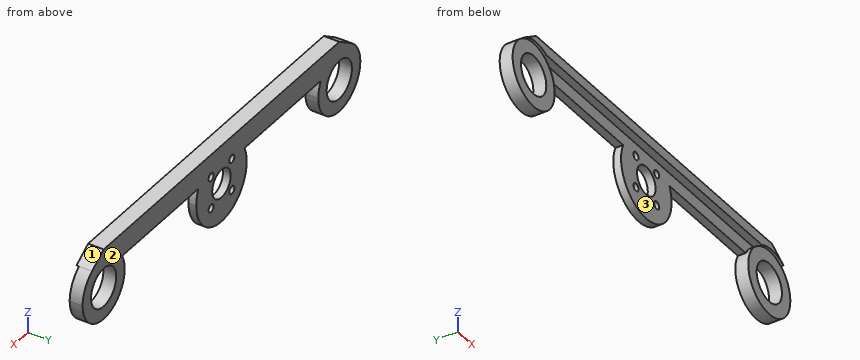
```python
from build123d import *

# Parameters (mm, degrees)
F0_R     = 1.5
F0_R_2   = 5.5
F1_DEPTH = 3
F0_R_3   = 7.5
F2_DEPTH = 5
F4_DEPTH = 3


with BuildPart() as f1:
    # F0 (on Front) → F1 (new body)
    with BuildSketch(Plane.XZ):
        with BuildLine():
            ThreePointArc((15, 0), (14.683594694, 3.0646446553), (13.7477270849, 6))
            ThreePointArc((13.7477270849, 6), (8.2158383626, 12.549900398), (0, 15))
            ThreePointArc((0, 15), (-8.2158383626, 12.549900398), (-13.7477270849, 6))
            ThreePointArc((-13.7477270849, 6), (-3.0646446553, -14.683594694), (15, 0))
        make_face()
        with Locations((-6.1518289963, -6.1518289963)):
            Circle(F0_R, mode=Mode.SUBTRACT)
        with Locations((6.1518289963, -6.1518289963)):
            Circle(F0_R, mode=Mode.SUBTRACT)
        with Locations((-6.1518289963, 6.1518289963)):
            Circle(F0_R, mode=Mode.SUBTRACT)
        Circle(F0_R_2, mode=Mode.SUBTRACT)
        with Locations((6.1518289963, 6.1518289963)):
            Circle(F0_R, mode=Mode.SUBTRACT)
        with BuildLine():
            ThreePointArc((59.0341439003, 6), (67.0016723737, 12.135074431), (76.9096349799, 10.4166666667))
            Line((76.9096349799, 10.4166666667), (70, 15))
            Line((70, 15), (0, 15))
            ThreePointArc((0, 15), (8.2158383626, 12.549900398), (13.7477270849, 6))
            Line((13.7477270849, 6), (59.0341439003, 6))
        make_face()
        with BuildLine():
            ThreePointArc((-13.7477270849, 6), (-8.2158383626, 12.549900398), (0, 15))
            Line((0, 15), (-70, 15))
            Line((-70, 15), (-76.9096349799, 10.4166666667))
            ThreePointArc((-76.9096349799, 10.4166666667), (-67.0016723737, 12.135074431), (-59.0341439003, 6))
            Line((-59.0341439003, 6), (-13.7477270849, 6))
        make_face()
    extrude(amount=F1_DEPTH)

    # F0 (on Front) → F2 (join)
    with BuildSketch(Plane.XZ):
        with BuildLine():
            ThreePointArc((59.0341439003, 6), (66.9034859315, -12.1103922572), (82.5, 0))
            ThreePointArc((82.5, 0), (81.0140918202, 5.9109881894), (76.9096349799, 10.4166666667))
            ThreePointArc((76.9096349799, 10.4166666667), (67.0016723737, 12.135074431), (59.0341439003, 6))
        make_face()
        with Locations((70, 0)):
            Circle(F0_R_3, mode=Mode.SUBTRACT)
        with BuildLine():
            ThreePointArc((-57.5, 0), (-57.8896077428, 3.0965140685), (-59.0341439003, 6))
            ThreePointArc((-59.0341439003, 6), (-67.0016723737, 12.135074431), (-76.9096349799, 10.4166666667))
            ThreePointArc((-76.9096349799, 10.4166666667), (-75.9109881894, -11.0140918202), (-57.5, 0))
        make_face()
        with Locations((-70, 0)):
            Circle(F0_R_3, mode=Mode.SUBTRACT)
    extrude(amount=F2_DEPTH)

    # F3 (on face) → F4 (join)
    with BuildSketch(Plane.XZ.offset(3)):
        with BuildLine():
            Line((0, 11), (64.0628289565, 11))
            ThreePointArc((64.0628289565, 11), (70.5670017384, 12.4871337395), (76.9096349799, 10.4166666667))
            Line((76.9096349799, 10.4166666667), (70, 15))
            Line((70, 15), (-70, 15))
            Line((-70, 15), (-76.9096349799, 10.4166666667))
            ThreePointArc((-76.9096349799, 10.4166666667), (-70.5670017384, 12.4871337395), (-64.0628289565, 11))
            Line((-64.0628289565, 11), (0, 11))
        make_face()
    extrude(amount=F4_DEPTH)


solid = f1.part
```
Can you work these out from the model? Positions are in its coordinate system, mm. Face numbers are marked on the shaded views. Give positions to 0.01 mm unless a question says otherwise; leave off trailing zeros. Order: outer loops, then holes, each group sorted by start corner. A loop starts at its lowest first (then second) coordinate and runs counter-clockwise, first axis right, second up. Notation, with made-up numbers: M 73.5,89 L 84.5,89 A21 cw 84.5,112 Z; hole C 45.25,43 d9. An arc over 180 degrees is marked long. Write item = value, one per line. Start each with the question number.
Q1. Suppose I cut it at A-A (x = 0). Write out the boundary of the cut face in (y, z), plus the area to 3 significant figures.
Q2. Suppose I cut it at D-D (z = -11). Write out the boundary of the cut face in (x, y).
Q3. We'd pull the mould along X, two halves only. Please class the marked faces 1, 2 and 3: pulls with the +X half, pulls with the -X half, needs draft (parallel to the pull), parting line crosses it, or undercut.
Q4. Will these pins go through, and if not, where does the flat tip stop? pin 1 Ø2.5 at (x, y) = (9, -4.5) entering from -Z; pin 2 Ø2 at (y, z) = (-2, -8) entering from -X; pin 3 Ø2.5 at (x, y) = (41.5, -1) entering from -Z; pin 4 Ø1.8 at (x, z) = (6.15, 6.15) entering from -Y (3 decimals).
Q5. Suppose I cut it at B-B (z = -3). Write out the boundary of the cut face in (x, y).
Q6. I need wall thicknesses on probe 1 along X at (y, z) = (-1.9, 0.5); probe 2 along Z at (x, y) = (-70, -2.25); probe 3 along X at (y, z) = (-0.9, -11.5). Which ranges of each line are inside material? Lowest first, please. Write a range as [from, to].
Q7. Suppose I cut it at C-C (x = -41.5). Write out the boundary of the cut face in (y, z).
Check result:
q1.outline = M -6,11 L -3,11 L -3,5.5 L 0,5.5 L 0,15 L -6,15 Z; M -3,-15 L 0,-15 L 0,-5.5 L -3,-5.5 Z
q1.area = 69.0 mm2
q2.outline = M -75.94,-5 L -64.06,-5 L -64.06,0 L -75.94,0 Z; M -10.2,-3 L 10.2,-3 L 10.2,0 L -10.2,0 Z; M 64.06,-5 L 75.94,-5 L 75.94,0 L 64.06,0 Z
q3.face_1 = pulls with the +X half
q3.face_2 = needs draft
q3.face_3 = undercut
q4.pin_1 = 11
q4.pin_2 = -80.36
q4.pin_3 = 6
q4.pin_4 = through
q5.outline = M -82.13,-5 L -76.87,-5 L -76.87,0 L -82.13,0 Z; M -63.13,-5 L -57.87,-5 L -57.87,0 L -63.13,0 Z; M -14.7,-3 L -4.61,-3 L -4.61,0 L -14.7,0 Z; M 4.61,-3 L 14.7,-3 L 14.7,0 L 4.61,0 Z; M 57.87,-5 L 63.13,-5 L 63.13,0 L 57.87,0 Z; M 76.87,-5 L 82.13,-5 L 82.13,0 L 76.87,0 Z
q6.probe_1 = [-82.49, -77.48], [-62.52, -57.51], [-14.99, -5.48], [5.48, 14.99], [57.51, 62.52], [77.48, 82.49]
q6.probe_2 = [-12.5, -7.5], [7.5, 15]
q6.probe_3 = [-74.9, -65.1], [-9.63, 9.63], [65.1, 74.9]
q7.outline = M -6,11 L -3,11 L -3,6 L 0,6 L 0,15 L -6,15 Z
